Autodesk Inventor part; units mm, degrees
ref_plane "YZ Plane" through (0, 0, 0) normal (1, 0, 0) x (0, 1, 0)
ref_plane "XZ Plane" through (0, 0, 0) normal (0, 1, 0) x (-1, 0, 0)
ref_plane "XY Plane" through (0, 0, 0) normal (0, 0, 1) x (1, 0, 0)
sketch "Szkic1" plane through (0, 0, 0) normal (0, 1, 0) x (-1, 0, 0)
  line L0 (0, 0) -> (20, 0)
  line L1 (20, 0) -> (20, 2)
  line L2 (20, 2) -> (0, 2)
  line L3 (0, 2) -> (0, 0)
  dimension "d20" = 20
  dimension "d21" = 2
sketch "Szkic5" plane through (0, 0, 0) normal (1, 0, 0) x (0, 1, 0)
  line L0 (0, 2) -> (0, 0) construction
  line L1 (0, 1) -> (14.1716, 1)
  line L2 (15.5858, 1.5858) -> (22.4142, 8.4142)
  line L3 (23.8284, 9) -> (30, 9)
  arc A0 (14.1716, 1) -> (15.5858, 1.5858) centre (14.1716, 3) ccw
  arc A1 (23.8284, 9) -> (22.4142, 8.4142) centre (23.8284, 7) ccw
  point P0 (15, 1)
  point P1 (23, 9)
  dimension "d22" = 15
  dimension "d23" = 8
  dimension "d24" = 30
  dimension "d25" = 45
  dimension "d27" = 2
sweep "Przeciągnięcie1" add profiles "Szkic1" path "Szkic5"
fillet "Zaokrąglenie1" radius 10 2 edges at (-20, 30, 9) (0, 30, 9)
sketch "Szkic2" plane through (-20, 23.8284, 10) normal (0, 0, 1) x (1, 0, 0)
  arc A0 (19.2381, 0) -> (0.7619, 0) centre (10, -3.8284) ccw
  point P0 (20, 26.1716)
  point P1 (0, 26.1716)
  point P2 (10, -6.8284)
  dimension "d29" = 3
hole "Otwór1" at (-10, 17, 10) direction (0, 0, -1) diameter 8.376 end through all
pattern_linear "Szyk prostokątny2" [suppressed]
equation "\"d12\" = Grubość"
equation "\"PromieńGięcia\" = Grubość"
equation "\"SzerokośćGięciaPodcięcia\" = Grubość"
equation "\"GłębokośćGięciaPodcięcia\" = 0.5 * Grubość"
equation "\"RozmiarPodcięciaNarożnika\" = 4 * Grubość"
equation "\"MinimalnaPozostałość\" = 2 * Grubość"
equation "\"PromieńPrzejścia\" = PromieńGięcia"
equation "\"Rozmiar_promienia_Jacobiego\" = Grubość"
equation "\"Wielk_odstępu\" = Grubość"
equation "\"d5\" = PromieńGięcia"
properties part number "Blaszka_do_ciągu" material "Aluminium 6061-AHC"
CAD build for the part. Positions are in the model's coordinates, mm. A direction names the side the tool comes from. Give positions to 0.01 mm unless a question says otherwise; leave off trailing zeros. Order: outer loops, then holes, each group sorted by start corner. A loop starts at its lowest first (then second) coordinate and runs counter-clockwise, first axis right, second up. Notation, with made-up numbers: (0, 10) -> (48, 10) arc R25 ccw to (48, 30) -> close; hole circle Ø4 at (16.5, 67.25). An arc over 180 degrees is marked (long way). Return JSON: item names as keys, results as strings.
Q1. Which spindle directions (+Z, -Z, +X, -X, +Y, -Y) get a long thin tool onto all of the face, cutting with end or side? Do faces 1 (the face through (-10, 7, 0)), 2 (the face through (-10, 7, 2)), 3 (the face through (-10, 26, 8)). Say none if no direction does.
Working result:
{"face 1": "-Z, +X, -X, +Y, -Y", "face 2": "+Z, +X, -X, -Y", "face 3": "-Z, +X, -X, +Y"}
Q2. Saw through at C-C (x = -1.75). Write the cut outline in (y, z).
Working result:
{"outline": "(0, 0) -> (14.17, 0) arc R3 ccw to (16.29, 0.88) -> (23.12, 7.71) arc R1 cw to (23.83, 8) -> (25.65, 8) -> (25.65, 10) -> (23.83, 10) arc R3 ccw to (21.71, 9.12) -> (14.88, 2.29) arc R1 cw to (14.17, 2) -> (0, 2) -> close"}
Q3. Saw through at D-D (y = 25). Write the cut outline in (x, z).
Working result:
{"outline": "(-18.66, 8) -> (-1.34, 8) -> (-1.34, 10) -> (-18.66, 10) -> close"}
Q4. Drill centre lines: line 1 (X direction, y = 17, z = 4.25); line 2 (Z direction, x = -8, y = 27.5); line 3 (Z direction, x = -1.5, y = 6). Where is each one in solid material? Low to high.
Working result:
{"line 1": "-20 to -14.19, -5.81 to 0", "line 2": "8 to 10", "line 3": "0 to 2"}
Q5. Mould opens along X. For faces 4 (the face through (0, 11.5, 1.8)), 5 (the face through (-12.362, 20.617, 8.031)), 6 (the face through (-13.396, 19.451, 4.613)), 7 (the face through (-20, 11, 1)) say: pulls with the +X half, pulls with the -X half, needs draft (parallel to the pull), parting line crosses it, or undercut.
Working result:
{"face 4": "pulls with the +X half", "face 5": "needs draft", "face 6": "undercut", "face 7": "pulls with the -X half"}
Q6. Saw through at B-B (x = -10). Write the cut outline in (y, z), then the cut area to 3 significant figures.
Working result:
{"outline": "(0, 0) -> (12.81, 0) -> (12.81, 2) -> (0, 2) -> close; (21.19, 5.77) -> (23.12, 7.71) arc R1 cw to (23.83, 8) -> (30, 8) -> (30, 10) -> (23.83, 10) arc R3 ccw to (21.71, 9.12) -> (21.19, 8.6) -> close", "area": "44.6 mm²"}
Q7. Saw through at A-A (y = 19). Write the cut outline in (x, z), then the cut area to 3 significant figures.
Working result:
{"outline": "(-20, 3.59) -> (-13.68, 3.59) -> (-13.68, 6.41) -> (-20, 6.41) -> close; (-6.32, 3.59) -> (0, 3.59) -> (0, 6.41) -> (-6.32, 6.41) -> close", "area": "35.8 mm²"}
Q8. Flat gauge pins, fed straight in: pin 1 (3 mm diameter, centred on x = -16.5, y = 27, fed in from -Z); pin 2 (11 mm diameter, centred on x = -10, y = 17, fed in from +Z); pin 3 (10 mm diameter, centred on x = -13.5, y = 20, fed in from -Z); pin 4 (1.5 mm diameter, centred on y = 10.5, z = 3, fed in from -X). Where does each tip first touch, or does it go through?
Working result:
{"pin 1": "z = 8", "pin 2": "z = 9.69", "pin 3": "z = 0.12", "pin 4": "through"}
